Read the model definition and answer for the solid it produces. Units are mm, in the model's axes. Face numbers are marked on the shaded views. A direction names the side the tool comes from. Give positions to 0.01 mm unless a question says otherwise; leave off trailing zeros. Loops run counter-clockwise (first coordinate to the right, second up) from the corner with the lowest first, then second, coordinate; pieces in that order, holes last. Notation, with made-up numbers: (23, 40.25) - (53, 40.25) arc R16 cw to (53, 62.25) - close; hole circle Ø2 at (20, 6). An arc over 180 degrees is marked (long way). Write each question's results on one line, items separated by ' | '. Start each with the question number.
Q1. Given pin 1 (0.6 mm diameter, centred on y = 2.5, z = -5.5, fed in from -X) (3 decimals); pin 2 (2 mm diameter, centred on y = 2.5, z = 1.5, fed in from -X) (3 decimals); pin 3 (1 mm diameter, centred on y = 3, z = 5.5, fed in from +X) (3 decimals); pin 4 (2 mm diameter, centred on x = -2.5, y = 0.5, fed in from -Z), each flat-ended and moving along its own axis, determine where each tip first touches the part or whether it passes through.
Q2. For the marked faces 1, 2, 3 and 4, determine the directions among +Z, -Z, +X, -X, +Y, -Y from which every point of the face is accessible in a straight line to the end or side of a thin tool.
Q3. The part is cut by section C-C, the plane y = 3.7. Write down the section's boundary in (x, z) (3 decimals), plus the area to 3 significant figures.
Q4. The part is cut by section D-D, the plane x = -1.25. Write down the section's boundary in (y, z).
Q5. Determine the mould class of the marked faces 5, 6, 7 and 8 for opening direction Y: +Y half, -Y half, draft (parallel to the pull), parting line (faces both ways), or undercut.
Q6. The part is cut by section B-B, the plane z = 1.5. Write down the section's boundary in (x, y) (3 decimals).
Q7. The part is cut by section A-A, the plane x = -3.5. Write down the section's boundary in (y, z).
Q8. Find the intervals of material crossed by line 1 (Y direction, x = 1.35, z = -1.5); line 2 (X direction, y = 1.25, z = -5) (3 decimals); line 3 (Z direction, x = 1.5, y = 3.4), in increasing order. Write a range as from..to.
Autodesk Inventor part; units mm, degrees
ref_plane "YZ Plane" through (0, 0, 0) normal (1, 0, 0) x (0, 1, 0)
ref_plane "XZ Plane" through (0, 0, 0) normal (0, 1, 0) x (-1, 0, 0)
ref_plane "XY Plane" through (0, 0, 0) normal (0, 0, 1) x (1, 0, 0)
sketch "Sketch1" plane through (0, 0, 0) normal (0, 1, 0) x (-1, 0, 0)
  line L0 (-2.055, 6.5) -> (2.055, 6.5)
  line L1 (2.055, 6.5) -> (2.055, -6.5)
  line L2 (2.055, -6.5) -> (-2.055, -6.5)
  line L3 (-2.055, -6.5) -> (-2.055, 6.5)
  line L4 (-2.055, 6.5) -> (2.055, -6.5) construction
  line L5 (2.055, 6.5) -> (-2.055, -6.5) construction
  point P0 (0, 0)
  dimension "d0" = 4.11
  dimension "d1" = 13
extrude "Extrusion1" add sketch "Sketch1" along normal blind 4
sketch "Sketch2" plane through (2.055, 0, 6.5) normal (1, 0, 0) x (0, 0, -1)
  line L0 (0, 0) -> (0, 4)
  line L1 (0, 2) -> (13, 2) construction
  line L2 (13, 0) -> (13, 4)
  line L3 (2, 0) -> (11, 0)
  line L4 (11, 4) -> (2, 4)
  arc A0 (2, 4) -> (2, 0) centre (2, 2) ccw
  arc A1 (11, 0) -> (11, 4) centre (11, 2) ccw
  line L5 (0, 4) -> (13, 4)
  line L6 (0, 0) -> (13, 0)
  point P0 (6.5, 0)
  point P1 (6.5, 2)
extrude "Extrusion2" cut sketch "Sketch2" against normal blind 2 contours L0 A0 L6 | L0 L5 A0 | A1 L2 L6 | L5 L2 A1
sketch "Sketch3" plane through (-2.055, 0, -6.5) normal (-1, 0, 0) x (0, 0, 1)
  arc A0 (2, 4) -> (0, 2) centre (2, 2) ccw
  line L0 (0, 0) -> (0, 4)
  line L1 (0, 4) -> (13, 4)
  arc A1 (0, 2) -> (2, 0) centre (2, 2) ccw
  arc A2 (2, 4) -> (2, 0) centre (2, 2) ccw
  line L2 (11, 4) -> (2, 4)
  arc A3 (11, 0) -> (11, 4) centre (11, 2) ccw
  line L3 (11, 0) -> (2, 0)
  line L4 (13, 0) -> (13, 4)
  line L5 (0, 0) -> (13, 0)
  point P0 (6.5, 0)
  point P1 (13, 2)
extrude "Extrusion3" cut sketch "Sketch3" against normal blind 1 contours A0 L0 L1 | A1 L5 L0 | L1 L4 A3 | L4 L5 A3
sketch "Sketch4" plane through (-2.055, 0, -4.5) normal (-1, 0, 0) x (0, 0, 1)
  arc A0 (0, 4) -> (-2, 2) centre (0, 2) ccw
  circle A1 centre (0, 2) radius 1.5
  arc A2 (11, 2) -> (9, 4) centre (9, 2) ccw
  circle A3 centre (9, 2) radius 1.5
  point P0 (4.5, 0)
  dimension "d8" = 3
  dimension "d9" = 3
mark "Mark1"
sketch "Sketch5" plane through (-2.055, 0, -4.5) normal (-1, 0, 0) x (0, 0, 1)
  circle A0 centre (3, 2) radius 1
  circle A1 centre (0, 2) radius 1.5
  circle A2 centre (9, 2) radius 1.5
  line L0 (0, 4) -> (9, 4)
  circle A3 centre (6, 2) radius 1
  point P0 (4.5, 0)
  dimension "d10" = 2
  dimension "d11" = 3
  dimension "d12" = 9
  dimension "d15" = 3
mark "Mark2"
sketch "Sketch6" plane through (-2.055, 2, -1.5) normal (-1, 0, 0) x (0, 0, 1)
  circle A0 centre (0, 0) radius 1
  circle A1 centre (0, 0) radius 0.5
  circle A2 centre (3, 0) radius 1
  circle A3 centre (3, 0) radius 0.5
  point P0 (1.5, -2)
  dimension "d20" = 1
  dimension "d21" = 1
extrude "Extrusion4" add sketch "Sketch6" along normal blind 2 contours A1 | A3
sketch "Sketch7" plane through (2.055, 0, 4.5) normal (1, 0, 0) x (0, 0, -1)
  circle A0 centre (0, 2) radius 1.5
  circle A1 centre (9, 2) radius 1.5
  point P0 (4.5, 0)
mark "Mark3"
sketch "Sketch8" plane through (2.055, 0, 4.5) normal (1, 0, 0) x (0, 0, -1)
  circle A0 centre (6, 2) radius 1
  circle A1 centre (3, 2) radius 1
  circle A2 centre (3, 2) radius 0.75
  circle A3 centre (6, 2) radius 0.75
  point P0 (4.5, 0)
  dimension "d24" = 1.5
  dimension "d25" = 1.5
extrude "Extrusion5" cut sketch "Sketch8" against normal blind 1 contours A2 | A3
sketch "Sketch9" plane through (1.055, 2, 1.5) normal (1, 0, 0) x (0, 0, -1)
  circle A0 centre (3, 0) radius 0.5
  circle A1 centre (0, 0) radius 0.5
  point P0 (1.5, -2)
extrude "Extrusion6" add sketch "Sketch9" along normal blind 2
fillet "Fillet1" radius 0.2 4 edges at (3.055, 2, 2) (3.055, 2, -1) (-4.055, 2, -2) (-4.055, 2, 1)
equation "\"d9\" = d8"
equation "\"d11\" = 0.333333 * d12"
equation "\"d15\" = d11"
equation "\"d21\" = d20"
equation "\"d25\" = d24"
properties part number "2_pin_no_ear_male"
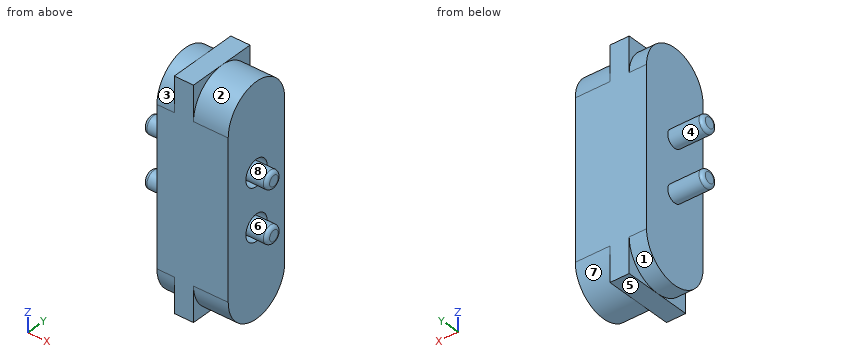
Check sheet entries:
1) pin 1: stops at x = -2.055 | pin 2: stops at x = -4.055 | pin 3: stops at x = 2.055 | pin 4: stops at z = -6.41
2) face 1: -Z, -X | face 2: +Z, +X | face 3: +Z, -X | face 4: -X
3) outline: (-2.055, -5.554) - (-1.055, -5.554) - (-1.055, -6.5) - (0.055, -6.5) - (0.055, -5.554) - (2.055, -5.554) - (2.055, 5.554) - (0.055, 5.554) - (0.055, 6.5) - (-1.055, 6.5) - (-1.055, 5.554) - (-2.055, 5.554) - close | area: 47.8 mm^2
4) outline: (0, -4.5) arc R2 ccw to (4, -4.5) - (4, 4.5) arc R2 ccw to (0, 4.5) - close
5) face 5: draft | face 6: undercut | face 7: parting line | face 8: undercut
6) outline: (-4.055, 1.7) arc R0.2 ccw to (-3.855, 1.5) - (-2.055, 1.5) - (-2.055, 0) - (2.055, 0) - (2.055, 1.25) - (1.055, 1.25) - (1.055, 1.5) - (2.855, 1.5) arc R0.2 ccw to (3.055, 1.7) - (3.055, 2.3) arc R0.2 ccw to (2.855, 2.5) - (1.055, 2.5) - (1.055, 2.75) - (2.055, 2.75) - (2.055, 4) - (-2.055, 4) - (-2.055, 2.5) - (-3.855, 2.5) arc R0.2 ccw to (-4.055, 2.3) - close
7) outline: circle Ø1 at (2, -1.5); circle Ø1 at (2, 1.5)
8) line 1: y = 0..1.25, 1.5..2.5, 2.75..4 | line 2: x = -2.055..2.055 | line 3: z = -5.93..5.93
